Build history of the part. All positions in model axes, mm. A direction names the side the tool comes from. Coordinates: 2 decimals unless noted, no trailing zeros. Order: outer loops, then holes, each group sorted by start corner. A loop starts at its lowest first (then second) coordinate and runs counter-clockwise, first axis right, second up. Notation, with made-up numbers: M 17,-18.5 L 44,-18.5 A19 ccw 44,11.5 Z; hole C 50.5,10 d5. An arc over 180 degrees is marked long. Use a Markdown table: item, result. Add a question column.
Autodesk Inventor part; units mm, degrees
ref_plane "YZ Plane" through (0, 0, 0) normal (1, 0, 0) x (0, 1, 0)
ref_plane "XZ Plane" through (0, 0, 0) normal (0, 1, 0) x (-1, 0, 0)
ref_plane "XY Plane" through (0, 0, 0) normal (0, 0, 1) x (1, 0, 0)
sketch "Sketch1" plane through (0, 0, 0) normal (0, 0, 1) x (1, 0, 0)
  circle A0 centre (0, 0) radius 30
  circle A1 centre (0, 100) radius 30
  line L0 (-20, 0) -> (20, 0)
  line L1 (20, 0) -> (20, 100)
  line L2 (20, 100) -> (-20, 100)
  line L3 (-20, 100) -> (-20, 0)
  point P0 (20, 77.6393)
  point P1 (-20, 77.6393)
  point P2 (-20, 22.3607)
  point P3 (20, 22.3607)
  dimension "d0" = 60
  dimension "d1" = 60
  dimension "d2" = 40
extrude "Extrusion1" add sketch "Sketch1" along normal blind 20
sketch "Sketch2" plane through (0, 0, 20) normal (0, 0, 1) x (1, 0, 0)
  circle A0 centre (0, 0) radius 10
  dimension "d5" = 20
extrude "Extrusion2" cut sketch "Sketch2" against normal blind 16
sketch "Sketch3" plane through (0, 0, 4) normal (0, 0, 1) x (1, 0, 0)
  circle A0 centre (0, 0) radius 1
  circle A1 centre (5, 0) radius 1
  circle A2 centre (-5, 0) radius 1
  dimension "d11" = 2
  dimension "d12" = 2
  dimension "d13" = 2
extrude "Extrusion3" cut sketch "Sketch3" against normal blind 28.45
sketch "Sketch4" plane through (0, 0, 0) normal (0, 0, -1) x (-1, 0, 0)
  line L0 (0, 100) -> (10, 100)
  line L1 (10, 100) -> (10, 70)
  line L2 (10, 70) -> (0, 70)
  line L3 (0, 70) -> (0, 100)
  line L4 (0, 100) -> (-10, 100)
  line L5 (-10, 100) -> (-10, 70)
  line L6 (-10, 70) -> (0, 70)
  line L7 (0, 70) -> (0, 100)
  line L8 (10, 100) -> (-10, 100)
  line L9 (-10, 100) -> (-10, 110.5)
  line L10 (-10, 110.5) -> (10, 110.5)
  line L11 (10, 110.5) -> (10, 100)
  point P0 (0, 0)
  dimension "d16" = 10
  dimension "d17" = 30
  dimension "d18" = 10
  dimension "d19" = 10.5
extrude "Extrusion4" cut sketch "Sketch4" against normal blind 16
sketch "Sketch5" plane through (0, 0, 0) normal (0, 0, -1) x (-1, 0, 0)
  line L0 (10, 110.5) -> (10, 70)
  line L1 (10, 110.5) -> (-10, 110.5)
  line L2 (-10, 110.5) -> (-10, 118.1)
  line L3 (-10, 118.1) -> (10, 118.1)
  line L4 (10, 118.1) -> (10, 110.5)
  line L5 (10, 70) -> (-10, 70)
  line L6 (-10, 70) -> (-10, 62.4)
  line L7 (-10, 62.4) -> (10, 62.4)
  line L8 (10, 62.4) -> (10, 70)
  line L9 (-10, 110.5) -> (10, 110.5)
  line L10 (10, 110.5) -> (-10, 110.5)
  line L11 (-10, 110.5) -> (-10, 114.6)
  line L12 (-10, 114.6) -> (10, 114.6)
  line L13 (10, 114.6) -> (10, 110.5)
  line L14 (10, 70) -> (-10, 70)
  line L15 (-10, 70) -> (-10, 65.9)
  line L16 (-10, 65.9) -> (10, 65.9)
  line L17 (10, 65.9) -> (10, 70)
  line L18 (0, 110.5) -> (5, 110.5)
  line L19 (5, 110.5) -> (5, 114.6)
  line L20 (5, 114.6) -> (0, 114.6)
  line L21 (0, 114.6) -> (0, 110.5)
  line L22 (0, 110.5) -> (-5, 110.5)
  line L23 (-5, 110.5) -> (-5, 114.6)
  line L24 (-5, 114.6) -> (0, 114.6)
  line L25 (0, 114.6) -> (0, 110.5)
  line L26 (0, 70) -> (5, 70)
  line L27 (5, 70) -> (5, 65.9)
  line L28 (5, 65.9) -> (0, 65.9)
  line L29 (0, 65.9) -> (0, 70)
  line L30 (0, 70) -> (-5, 70)
  line L31 (-5, 70) -> (-5, 65.9)
  line L32 (-5, 65.9) -> (0, 65.9)
  line L33 (0, 65.9) -> (0, 70)
  point P0 (0, 0)
  dimension "d22" = 7.6
  dimension "d23" = 7.6
  dimension "d24" = 4.1
  dimension "d25" = 4.1
  dimension "d26" = 5
  dimension "d27" = 5
  dimension "d28" = 5
  dimension "d29" = 5
extrude "Extrusion5" cut sketch "Sketch5" against normal blind 10
sketch "Sketch6" plane through (0, 0, 10) normal (0, 0, -1) x (-1, 0, 0)
  line L0 (10, 110.5) -> (10, 70)
  line L1 (-10, 62.4) -> (-10, 118.1)
  line L2 (10, 110.5) -> (-10, 110.5)
  line L3 (-10, 110.5) -> (-10, 114.6)
  line L4 (-10, 114.6) -> (10, 114.6)
  line L5 (10, 114.6) -> (10, 110.5)
  line L6 (10, 70) -> (-10, 70)
  line L7 (-10, 62.4) -> (-10, 70)
  line L8 (10, 70) -> (-10, 70)
  line L9 (-10, 70) -> (-10, 65.9)
  line L10 (-10, 65.9) -> (10, 65.9)
  line L11 (10, 65.9) -> (10, 70)
  line L12 (-10, 110.5) -> (10, 110.5)
  line L13 (0, 114.6) -> (5, 114.6)
  line L14 (5, 114.6) -> (5, 110.5)
  line L15 (5, 110.5) -> (0, 110.5)
  line L16 (0, 110.5) -> (0, 114.6)
  line L17 (0, 110.5) -> (-5, 110.5)
  line L18 (-5, 110.5) -> (-5, 114.6)
  line L19 (-5, 114.6) -> (0, 114.6)
  line L20 (0, 114.6) -> (0, 110.5)
  line L21 (0, 70) -> (5, 70)
  line L22 (5, 70) -> (5, 65.9)
  line L23 (5, 65.9) -> (0, 65.9)
  line L24 (0, 65.9) -> (0, 70)
  line L25 (0, 70) -> (-5, 70)
  line L26 (-5, 70) -> (-5, 65.9)
  line L27 (-5, 65.9) -> (0, 65.9)
  line L28 (0, 65.9) -> (0, 70)
  circle A0 centre (5, 114.6) radius 2.25
  circle A1 centre (-5, 114.6) radius 2.25
  circle A2 centre (5, 65.9) radius 2.25
  circle A3 centre (-5, 65.9) radius 2.25
  point P0 (0, 0)
  dimension "d32" = 4.1
  dimension "d33" = 4.1
  dimension "d34" = 5
  dimension "d35" = 5
  dimension "d36" = 4.5
  dimension "d37" = 4.5
  dimension "d38" = 4.5
  dimension "d39" = 4.5
extrude "Extrusion6" cut sketch "Sketch6" against normal blind 8 contours A0 L4 L14 | L14 L4 A0 | L4 A0 | A2 L10 L22 | L22 L10 A2 | A2 L10 | A1 L4 L18 | L18 L4 A1 | L4 A1 | A3 L10 L26 | L26 L10 A3 | A3 L10
thread "Thread1"
thread "Thread2"
thread "Thread3"
thread "Thread4"
sketch "Sketch7" plane through (0, 0, 20) normal (0, 0, 1) x (1, 0, 0)
  circle A0 centre (0, 100) radius 10
  point P0 (0, 0)
  dimension "d50" = 20
extrude "Extrusion7" cut sketch "Sketch7" against normal blind 4
sketch "Sketch8" plane through (0, 0, 0) normal (0, 0, -1) x (-1, 0, 0)
  line L0 (20, 77.6393) -> (20, 22.3607)
  arc A0 (20, 77.6393) -> (-20, 77.6393) centre (0, 100) ccw
  line L1 (20, 22.3607) -> (-20, 22.3607)
  line L2 (-20, 22.3607) -> (-20, 77.6393)
  line L3 (-20, 77.6393) -> (20, 77.6393)
  line L4 (20, 77.6393) -> (20, 22.3607)
  line L5 (10, 118.1) -> (10, 62.4)
  line L6 (10, 77.6393) -> (-10, 77.6393)
  line L7 (-10, 77.6393) -> (-10, 47.6393)
  line L8 (-10, 47.6393) -> (10, 47.6393)
  line L9 (10, 47.6393) -> (10, 77.6393)
  line L10 (-10, 22.3607) -> (10, 22.3607)
  line L11 (10, 22.3607) -> (10, 52.3607)
  line L12 (10, 52.3607) -> (-10, 52.3607)
  line L13 (-10, 52.3607) -> (-10, 22.3607)
  line L14 (20, 77.6393) -> (10, 52.3607)
  line L15 (10, 47.6393) -> (20, 22.3607)
  line L16 (-20, 77.6393) -> (-10, 52.3607)
  line L17 (-10, 47.6393) -> (-20, 22.3607)
  point P0 (0, 0)
  dimension "d53" = 20
  dimension "d54" = 30
  dimension "d55" = 30
extrude "Extrusion8" cut sketch "Sketch8" against normal blind 72.2 contours L0 L15 L9 L14 | L16 L7 L17 L2
sketch "Sketch9" plane through (0, 0, 20) normal (0, 0, 1) x (1, 0, 0)
  circle A0 centre (0, 0) radius 1
  circle A1 centre (0, 0) radius 10
extrude "Extrusion9" add sketch "Sketch9" against normal blind 20
sketch "Sketch10" plane through (0, 0, 0) normal (0, 0, -1) x (-1, 0, 0)
  circle A0 centre (0, 0) radius 1
  circle A1 centre (0, 0) radius 10
  dimension "d60" = 20
extrude "Extrusion10" cut sketch "Sketch10" against normal blind 16
sketch "Sketch11" plane through (0, 0, 16) normal (0, 0, -1) x (-1, 0, 0)
  circle A0 centre (0, 5) radius 1
  circle A1 centre (0, -5) radius 1
  point P0 (0, 0)
  dimension "d63" = 2
  dimension "d64" = 2
extrude "Extrusion11" cut sketch "Sketch11" against normal blind 22.1
chamfer "Chamfer2" distance 12 angle 45 1 edges at (10, 0, 0)
properties part number "2ndArm"
(1) Slice it at C-C on y = 114.6. Give the cut face in (x, z).
(2) Drop flat-ended pins along their axis: P1, Ø1.4, axis at y = 50.5, z = 6, coming from the +X side; P2, Ø5, axis at x = 22.5, z = 4, coming from the -Y side; P3, Ø4, axis at x = 5, y = 67.5, coming from the -Z side. Give the stop position or say it passes through.
(3) Slice it at B-B on z = 6.5. State how many separate pieces and enclosed holes the cut face has, and give its area (3 significant figures).
(4) Slice it at A-A on y = 92. Give the cut face in (x, z).
(5) Mould opens along Y. For faces 3 (the cylindrical face through (-1.013, 129.983, 9.86)), 4 (the flat face through (0, 51, 20)), 5 (the flat face through (-10, 50, 10)) say: released by +Y, released by -Y, zero draft, split by the parting line, or undercut.
(6) Slice it at D-D on y = 73. Give the cut face in (x, z), and give its area (3 significant figures).
(7) Which spindle directions (+Z, -Z, +X, -X, +Y, -Y) get a long thin tool onto all of the face, cutting with end or side? Do faces 1 (the flat face through (-2, 0, 16)), 2 (the cylindrical face through (1.013, -29.983, 9.86)). Say none if no direction does.
(8) Drill centre lines: line 1 along Y through (x, z) = (0, 14.8); line 2 along Y through (x, z) = (0, 17.4); line 3 along Y through (x, z) = (-5, 14.5). Where is each one in solid material? Low to high. Write a range as from..to.
Solutions:
| question | item | result |
|---|---|---|
| 1 | outline | M -26.21,0 L -10,0 L -10,10 L -7.25,10 L -7.25,18 L -2.75,18 L -2.75,10 L 2.75,10 L 2.75,18 L 7.25,18 L 7.25,10 L 10,10 L 10,0 L 26.21,0 L 26.21,20 L -26.21,20 Z |
| 2 | P1 | x = 10 |
| 2 | P2 | y = -22.36 |
| 2 | P3 | z = 10 |
| 3 | separate pieces | 1 |
| 3 | enclosed holes | 2 |
| 3 | area | 4,980 mm² |
| 4 | outline | M -28.91,0 L -10,0 L -10,16 L -6,16 L -6,20 L -28.91,20 Z; M 6,16 L 10,16 L 10,0 L 28.91,0 L 28.91,20 L 6,20 Z |
| 5 | face 3 | undercut |
| 5 | face 4 | zero draft |
| 5 | face 5 | undercut |
| 6 | outline | M -18.16,0 L -10,0 L -10,16 L 10,16 L 10,0 L 18.16,0 L 18.16,20 L -18.16,20 Z |
| 6 | area | 407 mm² |
| 7 | face 1 | -Z |
| 7 | face 2 | +Z, -Z |
| 8 | line 1 | -30..-10, 10..70, 110.5..130 |
| 8 | line 2 | -30..-6, -4..-1, 1..4, 6..90, 110..130 |
| 8 | line 3 | -29.58..-8.66, 8.66..63.65, 68.15..70, 110.5..112.35, 116.85..129.58 |
